Geometry check sheet. Reference: drawing and pictorial views, mm from the part's lowest x, y, z. A direction names the side the tool comes from. Coordinates: 2 decimals unless noted, no trailing zeros. Loops run counter-clockwise (first coordinate to the right, second up) from the corner with the lowest first, then second, coordinate; pieces in that order, holes last. Notation, with made-up numbers: M 56,-34 L 102,-34 A9 cw 102,-24 Z; hole C 45,64.5 d9. An arc over 180 degrees is marked long. Write item = value, one per line. Start each with the question number.
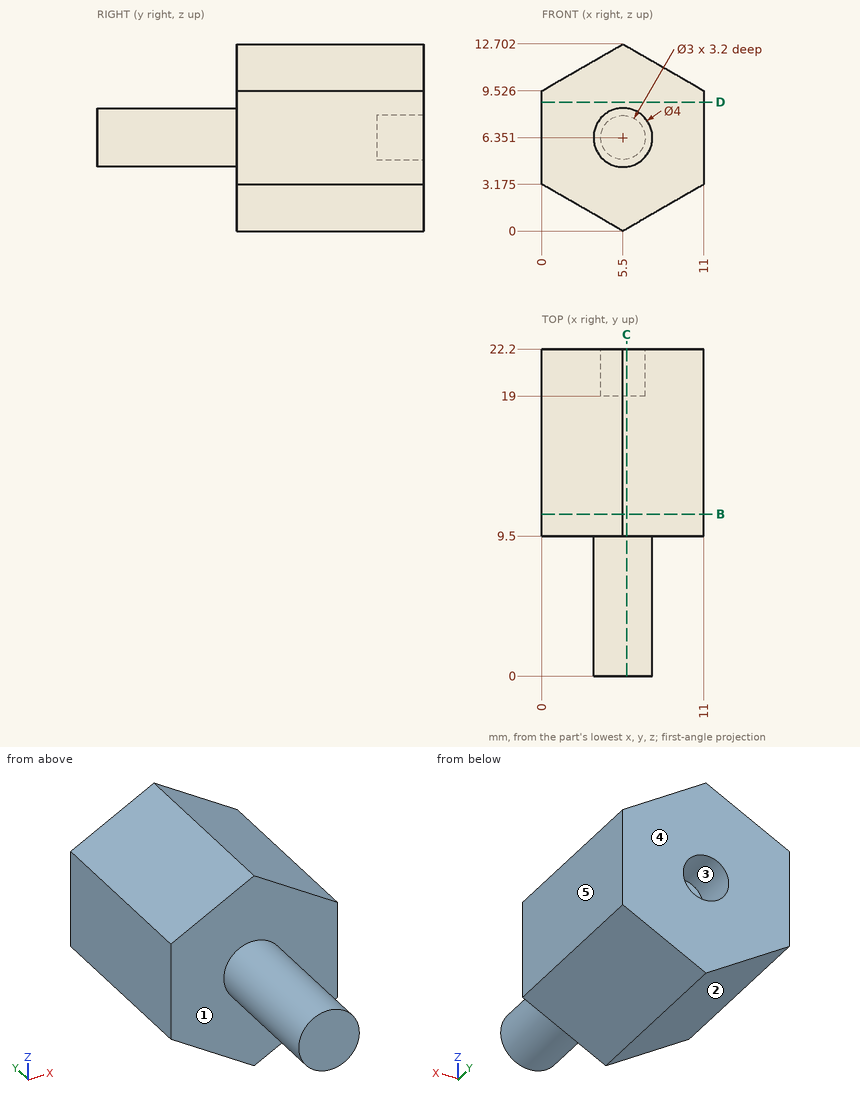
Q1. Scan lines: L1, parallel to Y at x = 3.5, z = 10.25; L2, parallel to Z at x = 6.25, y = 21; L3, parallel to Y at x = 6.5, z = 5.5. Record each from-to range of solid material in increasing order. Write a range as [from, to].
Q2. Sectioned sample at D-D on z = 8.75. Record the cut outline in (x, y), plus the area to 3 significant figures.
Q3. Gauge pin test, flat ends, axial feed: pin 1 (4 mm diameter, centred on x = 5.5, z = 6.35, fed in from +Y); pin 2 (0.9 mm diameter, centred on x = 5.5, z = 6.5, fed in from +Y); pin 3 (5 mm diameter, centred on x = 2.5, y = 12, fed in from -Z); pin 4 (6 mm diameter, centred on x = 7, y = 19.5, fed in from -Z). Record the tip position at first contact, or that the pin passes through.
Q4. Mould release check, pull along X, two halves, no side actions. Record for the marked faces 3, 4 and 5: +X half, -X half, draft (parallel to the pull), parting line (faces both ways), or undercut.
Q5. Set-up check for the marked faces 1 and 2: record each of +Z, -Z, +X, -X, +Y, -Y from which the full face is reachable in a straight line by a thin tool's end or side.
Q6. Sectioned sample at C-C on x = 5.75. Record the cut outline in (y, z) (1 decimal), plus the area to 3 significant figures.
Q7. Sectioned sample at B-B on y = 11. Record the cut outline in (x, z) (1 decimal).
Solutions:
q1.L1 = [9.5, 22.2]
q1.L2 = [0.43, 5.05], [7.65, 12.27]
q1.L3 = [0, 19]
q2.outline = M 0,9.5 L 11,9.5 L 11,22.2 L 0,22.2 Z
q2.area = 140 mm²
q3.pin_1 = 22.2
q3.pin_2 = 19
q3.pin_3 = 0.29
q3.pin_4 = 0
q4.face_3 = undercut
q4.face_4 = draft
q4.face_5 = +X half
q5.face_1 = -Y
q5.face_2 = -Z, -X, +Y, -Y
q6.outline = M 0,4.4 L 9.5,4.4 L 9.5,0.1 L 22.2,0.1 L 22.2,4.9 L 19,4.9 L 19,7.8 L 22.2,7.8 L 22.2,12.6 L 9.5,12.6 L 9.5,8.3 L 0,8.3 Z
q6.area = 186 mm²
q7.outline = M 0,3.2 L 5.5,0 L 11,3.2 L 11,9.5 L 5.5,12.7 L 0,9.5 Z
